Read the model definition and answer for the solid it produces. Units are mm, in the model's axes. A direction names the side the tool comes from. Give positions to 0.01 mm unless a question says otherwise; leave off trailing zeros. Loops run counter-clockwise (first coordinate to the right, second up) from the corner with the lowest first, then second, coordinate; pieces in that order, holes last. Notation, with made-up numbers: (-7, 23.25) -> (43, 23.25) arc R16 cw to (43, 40.25) -> close; hole circle Ø6 at (23.5, 77). An arc over 180 degrees is marked (long way). Answer as CSV lines item,"result". Start each with the question number.
```python
from build123d import *

# Parameters (mm, degrees)
F2_R         = 10.6813712462
F3_DEPTH     = 38.1
F4_S5_R      = 33.1123778597
F4_T6_DEPTH  = 17
F4_S11_R     = 33.1123778597
F4_T12_DEPTH = 17


# Not quite as in the source:
# - a fillet or chamfer that OpenCascade refuses, or shapes differently, is made with other operations: its cross-section is extruded or revolved along the edge and cut away or added


with BuildPart() as f1:
    # F0 (on Front) → F1 (revolve)
    with BuildSketch(Plane.XZ):
        Polygon((33.1123778597, 0), (0, 0), (0, -204.5256793499), (47.4873222411, -215.4780179262), (18.7374334782, -192.2043114901), (33.1123778597, -192.2043114901), (33.1123778597, -175.7757812738), (18.7374334782, -175.7757812738), (18.7374334782, -163.4543985128), (33.1123778597, -163.4543985128), (33.1123778597, -147.0258831978), (18.7374334782, -147.0258831978), (18.7374334782, -134.7045004368), (33.1123778597, -134.7045004368), align=None)
        Polygon((0, 204.5256793499), (0, 0), (33.1123778597, 0), (33.1123778597, 134.7045004368), (18.7374334782, 134.7045004368), (18.7374334782, 147.0258831978), (33.1123778597, 147.0258831978), (33.1123778597, 163.4543985128), (18.7374334782, 163.4543985128), (18.7374334782, 175.7757812738), (33.1123778597, 175.7757812738), (33.1123778597, 192.2043114901), (18.7374334782, 192.2043114901), (47.4873222411, 215.4780179262), align=None)
    revolve(axis=Axis((0, 0, -102.2628396749), (0, 0, -1)))

    # F2 (on Front) → F3 (join)
    with BuildSketch(Plane.XZ):
        with Locations((0, 113.5328859091)):
            Circle(F2_R)
        with Locations((0, -113.5328859091)):
            Circle(F2_R)
    extrude(amount=F3_DEPTH)

    # F4: chamfer of 5.08 on 2 edges, made by hand


with BuildPart() as f4_tool2:
    # F4_s3 → F4_t4 (revolve)
    with BuildSketch(Plane.XY.offset(113.5328859091)):
        Polygon((10.6813712462, -33.02), (5.6013712462, -38.1), (10.6813712462, -38.1), align=None)
    revolve(axis=Axis((0, -38.1, 113.5328859091), (0, -1, 0)))

    # F4_s5 → F4_t6 (cut, symmetric)
    with BuildSketch(Plane.XY.offset(113.5)):
        Circle(F4_S5_R)
    extrude(amount=F4_T6_DEPTH, both=True, mode=Mode.SUBTRACT)


with BuildPart() as f1_1:
    add(f1.part)

    # F4_t1: cut F4_tool2
    add(f4_tool2.part, mode=Mode.SUBTRACT)


with BuildPart() as f4_tool8:
    # F4_s9 → F4_t10 (revolve)
    with BuildSketch(Plane.XY.offset(-113.5328859091)):
        Polygon((10.6813712462, -33.02), (5.6013712462, -38.1), (10.6813712462, -38.1), align=None)
    revolve(axis=Axis((0, -38.1, -113.5328859091), (0, -1, 0)))

    # F4_s11 → F4_t12 (cut, symmetric)
    with BuildSketch(Plane.XY.offset(-113.5)):
        Circle(F4_S11_R)
    extrude(amount=F4_T12_DEPTH, both=True, mode=Mode.SUBTRACT)


with BuildPart() as f1_2:
    add(f1_1.part)

    # F4_t7: cut F4_tool8
    add(f4_tool8.part, mode=Mode.SUBTRACT)


solid = f1_2.part
```
(1) The mould has two halves that part along Z. Classify faces 1 (the face through (0, -38.1, -113)), 2 (the face through (-14, 14, 147.026)), 3 (the face through (-0.64, 2.9, -205.21)): pulls with the +Z half, pulls with the -Z half, needs draft (parallel to the pull), parting line crosses it, or undercut.
(2) A tool of negligible diameter and unlimited length cuts with its end or side. For faces 4 (the face through (10.68, -32.36, 113.33)), 5 (the face through (-0.761, -37.853, 119.331)), 6 (the face through (-10.68, -32.36, 113.73)), 7 (the face through (-14, 14, -163.454)), from which of +Z, -Z, +X, -X, +Y, -Y can it reach the whole face along a straight path? Write none if from no direction.
(3) Find the intervals of material crossed by line 1 along Z through (x, y) = (7, -34); line 2 along Y through (x, z) = (-0.5, -34.5); line 3 along Z through (x, y) = (4.5, -42), in increasing order. Write a range as from..to.
(4) Each of these flat-tipped pins is pushed along its axis until it touches: P1, Ø6, axis at x = 11, y = -7.5, coming from the +Z side; P2, Ø9, axis at x = -2, z = -113, coming from the -Y side; P3, Ø2, axis at x = 35, y = 12.5, coming from the -Z side. Where does it stop, or does it pass through?
(5) Find section B-B on z = -3. Write down the section's boundary in (x, y).
(6) Find section A-A on y = 29.5. Give the number of separate pieces and of enclosed holes in the cut face, then the cut area to 3 significant figures.
Answer block:
1,face 1,"undercut"
1,face 2,"undercut"
1,face 3,"pulls with the -Z half"
2,face 4,"+X, -Y"
2,face 5,"-Y"
2,face 6,"-X, -Y"
2,face 7,"none"
3,line 1,"z = -212.53..-205.14, -120.25..-106.82, 106.82..120.25, 205.14..212.53"
3,line 2,"y = -33.11..33.11"
3,line 3,"z = -214.27..-211.23, 211.23..214.27"
4,P1,"stops at z = 208.29"
4,P2,"stops at y = -38.1"
4,P3,"stops at z = -213.33"
5,outline,"circle Ø66.22 at (0, 0)"
6,separate pieces,"7"
6,enclosed holes,"0"
6,area,"11,100 mm2"
